The listing builds one solid part. Answer for the finished solid, in the listing's coordinates (mm). Give positions to 0.01 mm unless a question says otherwise; leave off trailing zeros. Write each loop counter-clockwise with the first axis right and the second up, starting at its lowest first coordinate (ties: lowest second). Pieces come first, ordered by that corner, then holes. Notation, with made-up numbers: (-26.5, 11) - (-12.5, 11) arc R23 ccw to (-12.5, 22) - close; hole circle Ø4 at (3, 86). An arc over 180 degrees is marked (long way). One line per item, written item: value. Start each with the question number.
from build123d import *

# Parameters (mm, degrees)
SKETCH1_W                        = 38.1
SKETCH1_H                        = 38.1
SKETCH1_W_2                      = 31.75
SKETCH1_H_2                      = 31.75
BOSS_EXTRUDE1_DEPTH              = 1101.725
F_10_0_1935_DIAMETER_HOLE1_D     = 4.9149
F_10_0_1935_DIAMETER_HOLE1_DEPTH = 3.175


with BuildPart() as part:
    # Sketch1 → Boss-Extrude1 (new body)
    with BuildSketch(Plane(origin=(0, 0, 0), x_dir=(0, 0, -1), z_dir=(1, 0, 0))):
        with Locations((19.05, 19.05)):
            Rectangle(SKETCH1_W, SKETCH1_H)
        with Locations((19.05, 19.05)):
            Rectangle(SKETCH1_W_2, SKETCH1_H_2, mode=Mode.SUBTRACT)
    extrude(amount=BOSS_EXTRUDE1_DEPTH)

    # #10 (0.1935) Diameter Hole1
    with Locations(Plane.XZ):
        with Locations((260.35, -19.05), (869.95, -19.05)):
            Hole(F_10_0_1935_DIAMETER_HOLE1_D / 2, depth=F_10_0_1935_DIAMETER_HOLE1_DEPTH)


solid = part.part
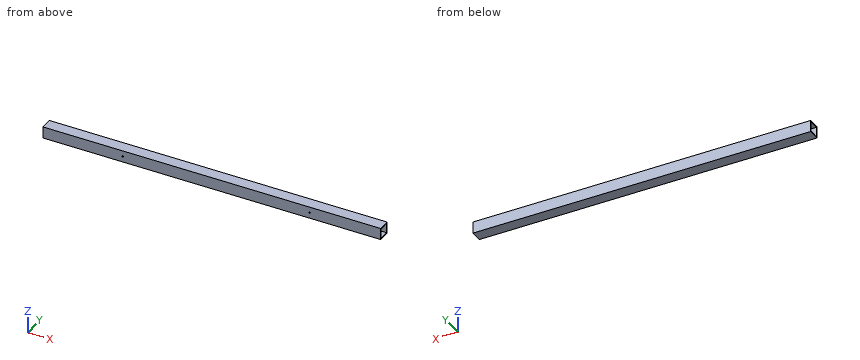
Item 1: Find section B-B on z = -28. Determine the outline of the cut face in (x, y) (3 decimals), plus the area to 3 significant figures.
Item 2: Straight lines are drawn through the part: line 1 along X through (y, z) = (2, -19) (3 decimals); line 2 along Y through (x, z) = (427, -21) (3 decimals); line 3 along Z through (x, y) = (1033.5, 30.5) (3 decimals). For each, find the intervals that lie inside material, in ascending order.
Item 3: Find section C-C on x = 1031. Determine the outline of the cut face in (y, z) (3 decimals), plus the area to 3 significant figures.
Item 4: This flat-tipped pin is pushed along its axis until it touches: pin 1 Ø6 at (x, y) = (415.5, 10.5) entering from +Z. Where does it stop, or does it pass through?
Item 5: Find section A-A on y = 27. Determine the outline of the cut face in (x, z) (3 decimals), plus the area to 3 significant figures.
Values:
1. outline: (0, 0) - (1101.725, 0) - (1101.725, 3.175) - (0, 3.175) - close; (0, 34.925) - (1101.725, 34.925) - (1101.725, 38.1) - (0, 38.1) - close
1. area: 7,000 mm^2
2. line 1: 0 to 257.893, 262.807 to 867.493, 872.407 to 1101.725
2. line 2: 0 to 3.175, 34.925 to 38.1
2. line 3: -38.1 to -34.925, -3.175 to 0
3. outline: (0, -38.1) - (38.1, -38.1) - (38.1, 0) - (0, 0) - close; hole (3.175, -34.925) - (34.925, -34.925) - (34.925, -3.175) - (3.175, -3.175) - close
3. area: 444 mm^2
4. pin 1: z = 0
5. outline: (0, -38.1) - (1101.725, -38.1) - (1101.725, -34.925) - (0, -34.925) - close; (0, -3.175) - (1101.725, -3.175) - (1101.725, 0) - (0, 0) - close
5. area: 7,000 mm^2
